Can you work these out from the model? Positions are in its coordinate system, mm. Face numbers are marked on the shaded views. A direction names the side the tool comes from. Give positions to 0.01 mm unless a question says otherwise; leave off trailing zeros. Order: outer loops, then holes, each group sorted by start corner. A loop starts at its lowest first (then second) coordinate and runs counter-clockwise, first axis right, second up.
Item 1: I want a section at C-C, the plane y = -21.7. Write out the boundary of the cut face in (x, z).
Item 2: I want a section at D-D, the plane x = 13. Write out the boundary of the cut face in (y, z), then the cut area to 3 significant figures.
Item 3: I'm going to push flat-ended pins straight in: pin 1 Ø1.5 at (y, z) = (-17.5, 1) entering from -X; pin 2 Ø0.9 at (y, z) = (-17.5, 1) entering from +X; pin 3 Ø1.5 at (x, z) = (0, 1.5) entering from +Y. Where does each tip first touch, or does it pass through?
Item 4: I want a section at B-B, the plane x = 1. Write out the boundary of the cut face in (y, z).
Item 5: If we mould it in two halves opening along Y, with no side actions, what happens to the marked faces 6, 7, 8 and 9? For each: +Y half, -Y half, draft (parallel to the pull), parting line (faces both ways), or undercut.
Item 6: Which directions (+Z, -Z, +X, -X, +Y, -Y) give clear straight access to the entire face, cutting with the end or side of a thin tool? Please do the marked faces 1, 2, 3, 4 and 5.
Item 7: If I drill on line 1 along Y through (x, z) = (2.5, 1.7); line 2 along Y through (x, z) = (13, 1.65); line 3 along X through (y, z) = (22.5, 2.3), over which ranges is the centre line in solid material (lowest first)?
Item 8: I want a section at A-A, the plane y = 15. Write out the boundary of the cut face in (x, z).
```python
from build123d import *

# Parameters (mm, degrees)
ESBO_O1_W                = 40.4
ESBO_O1_H                = 28.4
RESSALTO_EXTRUS_O1_DEPTH = 3
ESBO_O2_W                = 8
ESBO_O2_H                = 10.5
ESBO_O2_R                = 1.5
RESSALTO_EXTRUS_O2_DEPTH = 3
ESBO_O3_R                = 8.05
ESBO_O3_W                = 11
ESBO_O3_H                = 5.2
CORTE_EXTRUS_O1_DEPTH    = 33.048868935
FILETE1_R                = 1.5
FILETE2_R                = 1.5
FILETE3_R                = 1.5


with BuildPart() as part:
    # Esboço1 → Ressalto-extrusão1 (new body)
    with BuildSketch(Plane.XY):
        Rectangle(ESBO_O1_W, ESBO_O1_H)
    extrude(amount=RESSALTO_EXTRUS_O1_DEPTH)

    # Esboço2 → Ressalto-extrusão2 (add)
    # profile 1 of 4: a face of its own
    with BuildSketch(Plane.XY.offset(3)):
        with Locations((-13, -19.45)):
            Rectangle(ESBO_O2_W, ESBO_O2_H)
        with Locations((-13, -21.7)):
            Circle(ESBO_O2_R, mode=Mode.SUBTRACT)
    # profile 2 of 4: a face of its own
    with BuildSketch(Plane.XY.offset(3)):
        with Locations((13, -19.45)):
            Rectangle(ESBO_O2_W, ESBO_O2_H)
        with Locations((13, -21.7)):
            Circle(ESBO_O2_R, mode=Mode.SUBTRACT)
    # profile 3 of 4: a face of its own
    with BuildSketch(Plane.XY.offset(3)):
        with Locations((13, 19.45)):
            Rectangle(ESBO_O2_W, ESBO_O2_H)
        with Locations((13, 21.7)):
            Circle(ESBO_O2_R, mode=Mode.SUBTRACT)
    # profile 4 of 4: a face of its own
    with BuildSketch(Plane.XY.offset(3)):
        with Locations((-13, 19.45)):
            Rectangle(ESBO_O2_W, ESBO_O2_H)
        with Locations((-13, 21.7)):
            Circle(ESBO_O2_R, mode=Mode.SUBTRACT)
    extrude(amount=-RESSALTO_EXTRUS_O2_DEPTH)

    # Esboço3 → Corte-extrusão1 (cut, through all)
    with BuildSketch(Plane.XY.offset(3)):
        with Locations((-12.85, 0)):
            Circle(ESBO_O3_R)
        with Locations((12.85, 0)):
            Circle(ESBO_O3_R)
        with Locations((0, -7.6)):
            Rectangle(ESBO_O3_W, ESBO_O3_H)
        with Locations((0, 7.6)):
            Rectangle(ESBO_O3_W, ESBO_O3_H)
    extrude(amount=-CORTE_EXTRUS_O1_DEPTH, mode=Mode.SUBTRACT)

    # Filete1
    filete1_edges = [part.edges().sort_by_distance(p)[0] for p in [
        (-5.5, -5, 1.5),
        (5.5, -5, 1.5),
    ]]
    fillet(filete1_edges, radius=FILETE1_R)

    # Filete2
    filete2_edges = [part.edges().sort_by_distance(p)[0] for p in [
        (-5.5, -10.2, 1.5),
        (5.5, -10.2, 1.5),
    ]]
    fillet(filete2_edges, radius=FILETE2_R)

    # Filete3
    filete3_edges = [part.edges().sort_by_distance(p)[0] for p in [
        (5.5, 10.2, 1.5),
        (5.5, 5, 1.5),
        (-5.5, 5, 1.5),
        (-5.5, 10.2, 1.5),
    ]]
    fillet(filete3_edges, radius=FILETE3_R)


solid = part.part
```
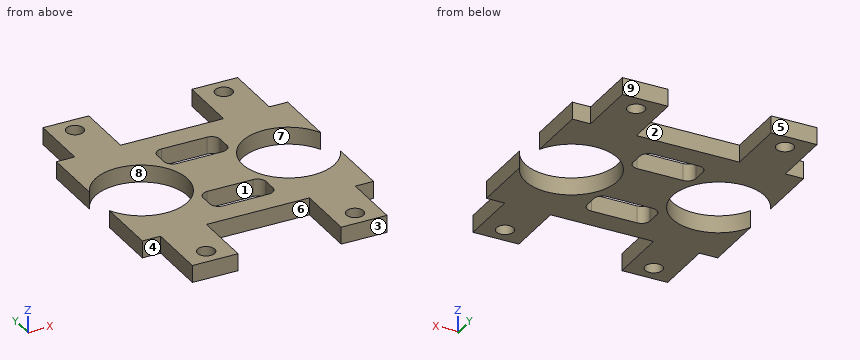
Results list:
1. outline: (-17, 0) - (-14.5, 0) - (-14.5, 3) - (-17, 3) - close; (-11.5, 0) - (-9, 0) - (-9, 3) - (-11.5, 3) - close; (9, 0) - (11.5, 0) - (11.5, 3) - (9, 3) - close; (14.5, 0) - (17, 0) - (17, 3) - (14.5, 3) - close
2. outline: (-24.7, 0) - (-23.2, 0) - (-23.2, 3) - (-24.7, 3) - close; (-20.2, 0) - (-8.05, 0) - (-8.05, 3) - (-20.2, 3) - close; (8.05, 0) - (20.2, 0) - (20.2, 3) - (8.05, 3) - close; (23.2, 0) - (24.7, 0) - (24.7, 3) - (23.2, 3) - close
2. area: 81.9 mm2
3. pin 1: stops at x = -17
3. pin 2: stops at x = 17
3. pin 3: stops at y = 14.2
4. outline: (-14.2, 0) - (-10.2, 0) - (-10.2, 3) - (-14.2, 3) - close; (-5, 0) - (5, 0) - (5, 3) - (-5, 3) - close; (10.2, 0) - (14.2, 0) - (14.2, 3) - (10.2, 3) - close
5. face 6: -Y half
5. face 7: undercut
5. face 8: undercut
5. face 9: +Y half
6. face 1: +Z, -Z
6. face 2: +Z, -Z, +Y
6. face 3: +Z, -Z, +X, -X, -Y
6. face 4: +Z, -Z, -X, -Y
6. face 5: +Z, -Z, +X, -X, +Y
7. line 1: y = -14.2 to -10.2, -5 to 5, 10.2 to 14.2
7. line 2: y = -24.7 to -23.2, -20.2 to -8.05, 8.05 to 20.2, 23.2 to 24.7
7. line 3: x = -17 to -14.27, -11.73 to -9, 9 to 11.73, 14.27 to 17
8. outline: (-17, 0) - (-9, 0) - (-9, 3) - (-17, 3) - close; (9, 0) - (17, 0) - (17, 3) - (9, 3) - close
